from build123d import *

# Parameters (mm, degrees)
SALIENTE_EXTRUIR1_DEPTH = 6
CROQUIS2_R              = 1.5
SALIENTE_EXTRUIR2_DEPTH = 6
CROQUIS3_R              = 1.5
CORTAR_EXTRUIR1_DEPTH   = 5.5


with BuildPart() as part:
    # Croquis1 → Saliente-Extruir1 (new body)
    with BuildSketch(Plane(origin=(0, 0, 0), x_dir=(1, 0, 0), z_dir=(0, 1, 0))):
        Polygon((0, 3.175426481), (-2.75, 1.58771324), (-2.75, -1.58771324), (0, -3.175426481), (2.75, -1.58771324), (2.75, 1.58771324), align=None)
    extrude(amount=SALIENTE_EXTRUIR1_DEPTH)

    # Croquis2 → Saliente-Extruir2 (add)
    with BuildSketch(Plane.XZ):
        Circle(CROQUIS2_R)
    extrude(amount=SALIENTE_EXTRUIR2_DEPTH)

    # Croquis3 → Cortar-Extruir1 (cut)
    with BuildSketch(Plane(origin=(0, 6, 0), x_dir=(1, 0, 0), z_dir=(0, 1, 0))):
        Circle(CROQUIS3_R)
    extrude(amount=-CORTAR_EXTRUIR1_DEPTH, mode=Mode.SUBTRACT)


solid = part.part
Can you work these out from the model? Positions are in its coordinate system, mm. A direction names the side the tool comes from. Give positions to 0.01 mm unless a question says otherwise; leave off trailing zeros. Write each loop counter-clockwise with the first axis right and the second up, starting at its lowest first coordinate (ties: lowest second). Pieces come first, ordered by that corner, then holes. Notation, with made-up numbers: M 56,9 L 75,9 A31 cw 75,42 Z; hole C -1,63.5 d6. An arc over 180 degrees is marked long. Answer in a Markdown table with one row per item. Add a question column.
Item 1: Imagine slicing it at C-C, the plane x = -0.65. Write out the boundary of the cut face in (y, z), plus the area to 3 significant figures.
Item 2: Imagine slicing it at A-A, the plane z = 0. Write out the boundary of the cut face in (x, y).
Item 3: Imagine slicing it at B-B, the plane y = -4.75. Write out the boundary of the cut face in (x, z).
Item 4: On a 3-axis mill with a long thin cutter (end or side, diameter ignored), from which of +Z, -Z, +X, -X, +Y, -Y can I reach the whole of each face in a straight line? I mean faces 4 (the cylindrical face through (-1.5, -2.96, 0.07)), 5 (the flat face through (1.394, 2.958, -2.37)), 6 (the cylindrical face through (-1.5, 3.29, -0.07)). Say none if no direction works.
Item 5: We'd pull the mould along X, two halves only. Please class faces 1 (the flat face through (-1.3, 6, 1.4)), 2 (the flat face through (-1.36, 2.96, -2.39)), 3 (the flat face through (0, 0.5, 0)): released by +X, released by -X, zero draft, split by the parting line, or undercut.
Item 6: Please list where these lines run through material, in increasing order: L1, parallel to X at y = 2.8, z = 0; L2, parallel to Y at x = 0.8, z = -1.75; L3, parallel to X at y = 1.75, z = 1.25.
Item 7: Imagine slicing it at D-D, the plane z = -1.75. Write out the boundary of the cut face in (x, y), plus the area to 3 significant figures.
Item 8: For pin 1 Ø1 at (y, z) = (-4, 0) entering from +X; pin 2 Ø1.5 at (x, z) = (0, 0) entering from +Y; pin 3 Ø1.5 at (x, y) = (1.5, 1.5) entering from +Z, each with a flat end and sliding along its axis, tell me the tip position at first contact or that it passes through.
Evaluation:
| question | item | result |
|---|---|---|
| 1 | outline | M -6,-1.35 L 0,-1.35 L 0,-2.8 L 6,-2.8 L 6,-1.35 L 0.5,-1.35 L 0.5,1.35 L 6,1.35 L 6,2.8 L 0,2.8 L 0,1.35 L -6,1.35 Z |
| 1 | area | 35.0 mm² |
| 2 | outline | M -2.75,0 L -1.5,0 L -1.5,-6 L 1.5,-6 L 1.5,0 L 2.75,0 L 2.75,6 L 1.5,6 L 1.5,0.5 L -1.5,0.5 L -1.5,6 L -2.75,6 Z |
| 3 | outline | C 0,0 d3 |
| 4 | face 4 | -Y |
| 4 | face 5 | -Z, +X, +Y, -Y |
| 4 | face 6 | +Y |
| 5 | face 1 | zero draft |
| 5 | face 2 | released by -X |
| 5 | face 3 | undercut |
| 6 | L1 | x = -2.75 to -1.5, 1.5 to 2.75 |
| 6 | L2 | y = 0 to 6 |
| 6 | L3 | x = -2.75 to -0.83, 0.83 to 2.75 |
| 7 | outline | M -2.47,0 L 2.47,0 L 2.47,6 L -2.47,6 Z |
| 7 | area | 29.6 mm² |
| 8 | pin 1 | stops at x = 1.5 |
| 8 | pin 2 | stops at y = 0.5 |
| 8 | pin 3 | stops at z = 2.74 |
